```python
from build123d import *

# Parameters (mm, degrees)
SKETCH1_W           = 3.048
SKETCH1_H           = 1.524
BOSS_EXTRUDE1_DEPTH = 1.524


with BuildPart() as part:
    # Sketch1 → Boss-Extrude1 (new body)
    with BuildSketch(Plane.XY):
        with BuildLine():
            Line((71.633966028, -1.524), (73.100370076, -1.524))
            Line((73.100370076, -1.524), (76.314988323, -3.549713839))
            ThreePointArc((76.314988323, -3.549713839), (76.575900985, -3.82622986), (76.670741226, -4.194389956))
            Line((76.670741226, -4.194389956), (76.670741226, -4.572894715))
            ThreePointArc((76.670741226, -4.572894715), (76.600333337, -4.892807754), (76.402120879, -5.153601627))
            Line((76.402120879, -5.153601627), (73.914078319, -7.267489978))
            ThreePointArc((73.914078319, -7.267489978), (73.683515458, -7.402025217), (73.420698665, -7.448783066))
            Line((73.420698665, -7.448783066), (67.716985472, -7.448783066))
            ThreePointArc((67.716985472, -7.448783066), (67.178170104, -7.225598434), (66.954985472, -6.686783066))
            Line((66.954985472, -6.686783066), (66.954985472, 5.162783066))
            ThreePointArc((66.954985472, 5.162783066), (67.178170104, 5.701598434), (67.716985472, 5.924783066))
            Line((67.716985472, 5.924783066), (73.420698665, 5.924783066))
            ThreePointArc((73.420698665, 5.924783066), (73.683515458, 5.878025217), (73.914078319, 5.743489978))
            Line((73.914078319, 5.743489978), (76.402120879, 3.629601627))
            ThreePointArc((76.402120879, 3.629601627), (76.600333337, 3.368807754), (76.670741226, 3.048894715))
            Line((76.670741226, 3.048894715), (76.670741226, 2.670389956))
            ThreePointArc((76.670741226, 2.670389956), (76.575900985, 2.30222986), (76.314988323, 2.025713839))
            Line((76.314988323, 2.025713839), (73.100370076, 0))
            Line((73.100370076, 0), (71.633966028, 0))
            Line((71.633966028, 0), (71.633966028, -1.524))
        make_face()
        with Locations((73.622741226, 2.859642336)):
            Rectangle(SKETCH1_W, SKETCH1_H, mode=Mode.SUBTRACT)
        with Locations((73.622741226, -4.383642336)):
            Rectangle(SKETCH1_W, SKETCH1_H, mode=Mode.SUBTRACT)
    extrude(amount=BOSS_EXTRUDE1_DEPTH)


solid = part.part
```
Source: CAD feature listing. Evaluate the final solid. Frame: model axes, mm. A direction names the side the tool comes from. Coordinates: 2 decimals unless noted, no trailing zeros. Order: outer loops, then holes, each group sorted by start corner. A loop starts at its lowest first (then second) coordinate and runs counter-clockwise, first axis right, second up. Notation, with made-up numbers: (18, 59) - (53, 59) arc R25 cw to (53, 94) - close; hole circle Ø10 at (73, -16). An arc over 180 degrees is marked (long way). One line per item, written item: value.
1) Contact query for a flat-ended pin moving along its axis: pin 1 (0.8 mm diameter, centred on y = -1, z = 1, fed in from +X). Output: stop coordinate, or through.
Computed values:
pin 1: stops at x = 71.63
2) Reachability of faces 4 (the face through (74.73, 1.027, 0.751)), 5 (the face through (71, -7.449, 1)), 6 (the face through (75.147, 3, 1)) from +Z, -Z, +X, -X, +Y, -Y: full face, straight path, thin tool, end or side. Return the list, or none.
Computed values:
face 4: +Z, -Z, +X
face 5: +Z, -Z, +X, -X, -Y
face 6: +Z, -Z
3) Cut plane B-B on z = 0.95. Output: boundary loops of the cut face in (x, y).
Computed values:
outline: (66.95, -6.69) arc R0.76 ccw to (67.72, -7.45) - (73.42, -7.45) arc R0.76 ccw to (73.91, -7.27) - (76.4, -5.15) arc R0.76 ccw to (76.67, -4.57) - (76.67, -4.19) arc R0.76 ccw to (76.31, -3.55) - (73.1, -1.52) - (71.63, -1.52) - (71.63, 0) - (73.1, 0) - (76.31, 2.03) arc R0.76 ccw to (76.67, 2.67) - (76.67, 3.05) arc R0.76 ccw to (76.4, 3.63) - (73.91, 5.74) arc R0.76 ccw to (73.42, 5.92) - (67.72, 5.92) arc R0.76 ccw to (66.95, 5.16) - close; hole (72.1, -5.15) - (75.15, -5.15) - (75.15, -3.62) - (72.1, -3.62) - close; hole (72.1, 2.1) - (75.15, 2.1) - (75.15, 3.62) - (72.1, 3.62) - close
4) Ray query, line 1 (Y direction, x = 72.75, z = 0.8); line 2 (Y direction, x = 74.5, z = 1.4); line 3 (X direction, y = 3, z = 0.95). Return the intervals inside material, ascending. Write a range as [from, to].
Computed values:
line 1: y = [-7.45, -5.15], [-3.62, -1.52], [0, 2.1], [3.62, 5.92]
line 2: y = [-6.77, -5.15], [-3.62, -2.41], [0.88, 2.1], [3.62, 5.25]
line 3: x = [66.95, 72.1], [75.15, 76.67]
5) Mould query, pull axis Y, two halves, no side actions, for faces 1 (the face through (71, 5.925, 1)), 2 (the face through (72, 0, 1)), 3 (the face through (71, -1, 0)). Classes: released by +Y, released by -Y, zero draft, split by the parting line, or undercut.
Computed values:
face 1: released by +Y
face 2: undercut
face 3: zero draft
6) Cut plane D-D on y = -1.25. Output: boundary loops of the cut face in (x, z), plus the area to 3 significant figures.
Computed values:
outline: (66.95, 0) - (71.63, 0) - (71.63, 1.52) - (66.95, 1.52) - close
area: 7.13 mm^2
7) Cut plane A-A on x = 72.25. Output: boundary loops of the cut face in (y, z).
Computed values:
outline: (-7.45, 0) - (-5.15, 0) - (-5.15, 1.52) - (-7.45, 1.52) - close; (-3.62, 0) - (-1.52, 0) - (-1.52, 1.52) - (-3.62, 1.52) - close; (0, 0) - (2.1, 0) - (2.1, 1.52) - (0, 1.52) - close; (3.62, 0) - (5.92, 0) - (5.92, 1.52) - (3.62, 1.52) - close
8) Cut plane C-C on x = 75.5. Output: boundary loops of the cut face in (y, z).
Computed values:
outline: (-5.92, 0) - (-3.04, 0) - (-3.04, 1.52) - (-5.92, 1.52) - close; (1.51, 0) - (4.4, 0) - (4.4, 1.52) - (1.51, 1.52) - close
